For this review, take the finished solid that the model builds, in its own axes (mm). A direction names the side the tool comes from. Round coordinates to 2 decimals unless told otherwise and drop trailing zeros. Write each loop counter-clockwise with the first axis right and the second up, starting at its lowest first coordinate (ties: lowest second). Pieces come first, ordered by that corner, then holes. Notation, with made-up numbers: (4, 7.5) - (21, 7.5) arc R34 ccw to (21, 40.5) - close; hole circle Ø10 at (-38.75, -29.5). An arc over 180 degrees is marked (long way). One line per item, written item: value. Start each with the question number.
Q1. For probe 1 along X at (y, z) = (-15.25, 0.5); probe 2 along X at (y, z) = (-23.5, 8); probe 3 along X at (y, z) = (-5.5, 22), list the stretches that pass through material, from the lowest coordinate up.
Q2. Add section B-B on x = 4. Write out the cut boundary in (y, z), and give its area (3 significant figures).
Q3. Add section A-A on z = 0. Write out the cut boundary in (x, y), and give its area (3 significant figures).
Q4. Tool access review of faces 1 (the face through (5, -12, 23)), 2 (the face through (-5, -12, 23)), 3 (the face through (12.13, -12.32, -10.03)): name each direction out of +Z, -Z, +X, -X, +Y, -Y from which nothing blocks a thin tool from reaching the whole face with its end or side.
Q5. Mouldability with a two-part tool opening along Z and no side actions: class faces 4 (the face through (0, -12, 26.572)), 5 (the face through (-17.474, -12.325, 9.73)), 6 (the face through (-9, 0, 11)), 7 (the face through (-12.13, -12.32, -10.03)) as +Z half, -Z half, draft (parallel to the pull), parting line (faces both ways), or undercut.
Q6. Add section C-C on z = 6. Write out the cut boundary in (x, y), and give its area (3 significant figures).
Q7. Add section D-D on z = 18. Write out the cut boundary in (x, y), and give its area (3 significant figures).
Q8. Clearance check with flat-ended pins moving along their axes: pin 1 Ø5 at (y, z) = (-20, 0) entering from -X; pin 2 Ø1 at (y, z) = (-15.5, 3.5) entering from -X; pin 3 Ø6 at (x, y) = (-9.5, -8.5) entering from -Z. State where each tip first meets the part, or that it passes through.
```python
from build123d import *

# Parameters (mm, degrees)
F1_DEPTH = 25
F3_R     = 5


# Not quite as in the source:
# - a feature names something its author has since deleted; it is built from what else it names


with BuildPart() as f1:
    # F0 (on Front) → F1 (new body)
    with BuildSketch(Plane.XZ):
        with BuildLine():
            ThreePointArc((11.897, -13.5710131507), (19.9295853554, -17.8647399206), (17.8635986234, -8.9939893385))
            ThreePointArc((17.8635986234, -8.9939893385), (18.2138113493, 8.2617840768), (5, 19.364916731))
            Line((5, 19.364916731), (5, 26.5722312033))
            Line((5, 26.5722312033), (0, 26.5722312033))
            Line((0, 26.5722312033), (0, 20))
            Line((0, 20), (0, 14))
            ThreePointArc((0, 14), (12.0042367313, 7.2040475081), (12.3541559587, -6.5859570715))
            Line((12.3541559587, -6.5859570715), (11.897, -13.5710131507))
        make_face()
    extrude(amount=F1_DEPTH)

    # F2: F1 across plane


with BuildPart() as f1_1:
    add(f1.part)
    add(f1.part.mirror(Plane.YZ))

    # F3
    f3_edges = [f1_1.edges().sort_by_distance(p)[0] for p in [
        (-17.863599, -12.5, -8.993989),
        (17.863599, -12.5, -8.993989),
        (0, -25, 26.572231),
        (0, 0, 26.572231),
    ]]
    fillet(f3_edges, radius=F3_R)


solid = f1_1.part
```
Result set:
1. probe 1: x = -19.99 to -13.99, 13.99 to 19.99
1. probe 2: x = -18.33 to -11.49, 11.49 to 18.33
1. probe 3: x = -5 to 5
2. outline: (-25, 13.42) - (0, 13.42) - (0, 21.57) arc R5 ccw to (-5, 26.57) - (-20, 26.57) arc R5 ccw to (-25, 21.57) - close
2. area: 318 mm^2
3. outline: (-20, -25) - (-14, -25) - (-14, 0) - (-20, 0) - close; (14, -25) - (20, -25) - (20, 0) - (14, 0) - close
3. area: 300 mm^2
4. face 1: +Z, +X, +Y, -Y
4. face 2: +Z, -X, +Y, -Y
4. face 3: +Y, -Y
5. face 4: +Z half
5. face 5: undercut
5. face 6: draft
5. face 7: undercut
6. outline: (-19.08, -25) - (-12.65, -25) - (-12.65, 0) - (-19.08, 0) - close; (12.65, -25) - (19.08, -25) - (19.08, 0) - (12.65, 0) - close
6. area: 321 mm^2
7. outline: (-8.72, -25) - (8.72, -25) - (8.72, 0) - (-8.72, 0) - close
7. area: 436 mm^2
8. pin 1: stops at x = -20
8. pin 2: stops at x = -19.77
8. pin 3: stops at z = -16.3
